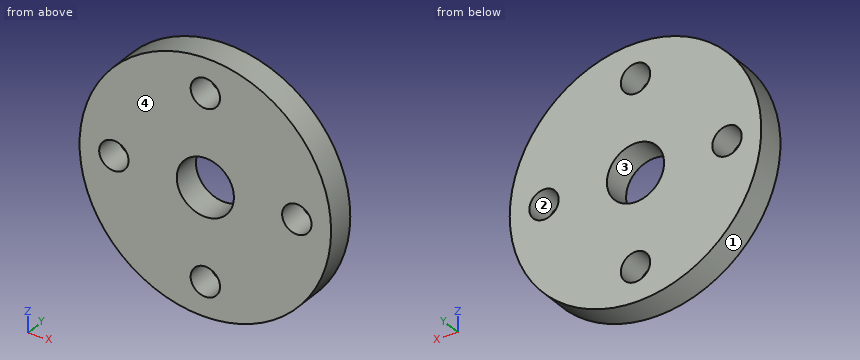
from build123d import *

# Parameters (mm, degrees)
SKETCH1_R           = 13.97
BOSS_EXTRUDE1_DEPTH = 3.175
SKETCH2_R           = 3.175
CUT_EXTRUDE1_DEPTH  = 3.175
CIRPATTERN1_COUNT   = 4


with BuildPart() as part:
    # Sketch1 → Boss-Extrude1 (new body)
    with BuildSketch(Plane(origin=(0, 0, 0), x_dir=(1, 0, 0), z_dir=(0, 1, 0))):
        Circle(SKETCH1_R)
    extrude(amount=BOSS_EXTRUDE1_DEPTH)

    # Sketch2 → Cut-Extrude1 (cut)
    with BuildSketch(Plane(origin=(0, 3.175, 0), x_dir=(1, 0, 0), z_dir=(0, 1, 0))):
        Circle(SKETCH2_R)
    extrude(amount=-CUT_EXTRUDE1_DEPTH, mode=Mode.SUBTRACT)

    # Sketch3 → #4 Clearance Hole1 (revolve, cut)
    with BuildSketch(Plane(origin=(0, 3.175, -10.16), x_dir=(0, 0, 1), z_dir=(1, 0, 0))):
        Polygon((0, 0), (0, 11.140574487), (1.63195, 10.16), (1.63195, 0), align=None)
    f_4_clearance_hole1 = revolve(axis=Axis((0, 9.525, -10.16), (0, -1, 0)), mode=Mode.SUBTRACT)

    # CirPattern1: #4 Clearance Hole1 ×4 about axis
    cirpattern1_axis = Axis((0, 0, 0), (0, 1, 0))
    for i in range(1, CIRPATTERN1_COUNT):
        add(f_4_clearance_hole1.rotate(cirpattern1_axis, i * 360 / CIRPATTERN1_COUNT), mode=Mode.SUBTRACT)


solid = part.part
Verification items for the finished model (mm, model axes). Face numbers are marked on the shaded views. Coordinates: 2 decimals unless noted, no trailing zeros. Loops run counter-clockwise (first coordinate to the right, second up) from the corner with the lowest first, then second, coordinate; pieces in that order, holes last. Notation, with made-up numbers: (15, -3.5) -> (30, -3.5) arc R18 cw to (30, 24.5) -> close; hole circle Ø1 at (-10.5, 74). An arc over 180 degrees is marked (long way). Answer as a JSON object with one key per item and string values. Group by question number.
Item 1: Sectioned sample at C-C on y = 0.5. Record the boundary of the cut face in (x, z) (3 decimals).
Item 2: Depth check by flat-ended pin: pin 1 (3 mm diameter, centred on x = -10.16, z = 0, fed in from +Y). Enter the tip coordinate at first touch or a pass-through.
Item 3: Mould release check, pull along X, two halves, no side actions. Record for the marked faces 1, 2, 3 and 4: +X half, -X half, draft (parallel to the pull), parting line (faces both ways), or undercut.
Item 4: Sectioned sample at D-D on x = -10.16. Record the boundary of the cut face in (y, z) (3 decimals).
Item 5: Sectioned sample at A-A on z = 0. Record the boundary of the cut face in (x, y) (3 decimals), plus the area to 3 significant figures.
Item 6: Sectioned sample at B-B on x = 0. Record the boundary of the cut face in (y, z) (3 decimals), plus the area to 3 significant figures.
Item 7: Scan lines: probe 1 along Z at (x, y) = (0, 2.2) (3 decimals); probe 2 along Z at (x, y) = (10.5, 2.7); probe 3 along Z at (x, y) = (9, 2). Record each from-to range of solid material in increasing order.
Evaluation:
{
 "1": {"outline": "circle Ø27.94 at (0, 0); hole circle Ø3.264 at (-10.16, 0); hole circle Ø6.35 at (0, 0); hole circle Ø3.264 at (0, -10.16); hole circle Ø3.264 at (0, 10.16); hole circle Ø3.264 at (10.16, 0)"},
 "2": {"pin 1": "passes through"},
 "3": {"face 1": "parting line", "face 2": "undercut", "face 3": "undercut", "face 4": "draft"},
 "4": {"outline": "(0, -9.588) -> (3.175, -9.588) -> (3.175, -1.632) -> (0, -1.632) -> close; (0, 1.632) -> (3.175, 1.632) -> (3.175, 9.588) -> (0, 9.588) -> close"},
 "5": {"outline": "(-13.97, 0) -> (-11.792, 0) -> (-11.792, 3.175) -> (-13.97, 3.175) -> close; (-8.528, 0) -> (-3.175, 0) -> (-3.175, 3.175) -> (-8.528, 3.175) -> close; (3.175, 0) -> (8.528, 0) -> (8.528, 3.175) -> (3.175, 3.175) -> close; (11.792, 0) -> (13.97, 0) -> (13.97, 3.175) -> (11.792, 3.175) -> close", "area": "47.8 mm²"},
 "6": {"outline": "(0, -13.97) -> (3.175, -13.97) -> (3.175, -11.792) -> (0, -11.792) -> close; (0, -8.528) -> (3.175, -8.528) -> (3.175, -3.175) -> (0, -3.175) -> close; (0, 3.175) -> (3.175, 3.175) -> (3.175, 8.528) -> (0, 8.528) -> close; (0, 11.792) -> (3.175, 11.792) -> (3.175, 13.97) -> (0, 13.97) -> close", "area": "47.8 mm²"},
 "7": {"probe 1": "z = -13.97 to -11.792, -8.528 to -3.175, 3.175 to 8.528, 11.792 to 13.97", "probe 2": "z = -9.21 to -1.6, 1.6 to 9.21", "probe 3": "z = -10.68 to -1.15, 1.15 to 10.68"}
}
